Model file for the job. Use its own axes, mm. A direction names the side the tool comes from. Coordinates: 2 decimals unless noted, no trailing zeros. Write each loop counter-clockwise with the first axis right and the second up, starting at its lowest first coordinate (ties: lowest second). Pieces come first, ordered by that corner, then holes. Notation, with made-up numbers: M 27,-25.75 L 39,-25.75 A10 ccw 39,-9.75 Z; hole C 41.5,11 d7. An arc over 180 degrees is marked long. One line per question, with ' | ' between items. Start each with the question number.
(1) Two-plate mould, pull along Z, no slides. Class faces 1 (the face through (-0.423, 2.134, 6.778)), 2 (the face through (39, 19.05, 12)): +Z half, -Z half, draft (parallel to the pull), parting line (faces both ways), or undercut.
(2) Tool access for faces 3 (the face through (39, -19.05, 12)), 4 (the face through (17, -3.81, 1)), 5 (the face through (-13.247, 2.134, -0.143)): list every direction of +Z, -Z, +X, -X, +Y, -Y with a clear straight run to the whole face (end or side of a thin tool).
(3) Wall check: probe 1 along Z at (x, y) = (0, 0); probe 2 along Z at (x, y) = (0, 2). Give the ranges that are in metal, low to high.
(4) Flat gauge pins, fed straight in: pin 1 Ø4 at (x, z) = (0, -10) entering from -Y; pin 2 Ø3 at (x, y) = (41, 1) entering from -Z; pin 3 Ø6 at (x, z) = (0, 10) entering from +Y; pin 4 Ø2.5 at (x, z) = (10, 0) entering from +Y. Where does each tip first touch, or does it go through?
(5) Cut at D-D (x = -35.5). Write the cut outline in (y, z).
(6) Cut at A-A (z = 0). Count the separate pieces of the cut face and the enclosed holes in it, plus the area to 3 significant figures.
(7) Cut at C-C (y = 15.5). Write the cut outline in (x, z), plus the area to 3 significant figures.
(8) Cut at B-B (x = 10). Write the cut outline in (y, z), plus the area to 3 significant figures.
from build123d import *

# Parameters (mm, degrees)
SKETCH1_R                                           = 59.69
BOSS_EXTRUDE1_DEPTH                                 = 19.05
BOSS_EXTRUDE1_DEPTH_BACK                            = 19.05
SKETCH2_R                                           = 40.64
CUT_EXTRUDE2_DEPTH                                  = 15.24
SKETCH13_R                                          = 40.64
CUT_EXTRUDE7_DEPTH                                  = 15.24
SKETCH7_R                                           = 4
CUT_EXTRUDE6_DEPTH                                  = 25
SKETCH6_R                                           = 1.7
CUT_EXTRUDE5_DEPTH                                  = 10
CIRPATTERN2_COUNT                                   = 4
CBORE_FOR_M3_HEX_SOCKET_HEAD_CAP_SCREW1_D           = 3.4
CBORE_FOR_M3_HEX_SOCKET_HEAD_CAP_SCREW1_DEPTH       = 5
CBORE_FOR_M3_HEX_SOCKET_HEAD_CAP_SCREW1_CBORE_D     = 6.5
CBORE_FOR_M3_HEX_SOCKET_HEAD_CAP_SCREW1_CBORE_DEPTH = 3.4
CBORE_FOR_M3_HEX_SOCKET_HEAD_CAP_SCREW1_TIP         = 1.021463052
SKETCH14_R                                          = 15
CUT_EXTRUDE8_DEPTH                                  = 2


with BuildPart() as part:
    # Sketch1 → Boss-Extrude1 (new body, two sides)
    with BuildSketch(Plane(origin=(0, 0, 0), x_dir=(1, 0, 0), z_dir=(0, 1, 0))) as boss_extrude1_sk:
        Circle(SKETCH1_R)
    extrude(amount=BOSS_EXTRUDE1_DEPTH)
    extrude(boss_extrude1_sk.sketch, amount=-BOSS_EXTRUDE1_DEPTH_BACK)

    # Sketch2 → Cut-Extrude2 (cut)
    with BuildSketch(Plane.XZ.offset(19.05)):
        Circle(SKETCH2_R)
    extrude(amount=-CUT_EXTRUDE2_DEPTH, mode=Mode.SUBTRACT)

    # Sketch13 → Cut-Extrude7 (cut)
    with BuildSketch(Plane(origin=(0, 19.05, 0), x_dir=(1, 0, 0), z_dir=(0, 1, 0))):
        Circle(SKETCH13_R)
    extrude(amount=-CUT_EXTRUDE7_DEPTH, mode=Mode.SUBTRACT)

    # Sketch7 → Cut-Extrude6 (cut)
    with BuildSketch(Plane(origin=(0, 3.81, 0), x_dir=(1, 0, 0), z_dir=(0, 1, 0))):
        Circle(SKETCH7_R)
    cut_extrude6 = extrude(amount=-CUT_EXTRUDE6_DEPTH, mode=Mode.SUBTRACT)

    # Sketch6 → Cut-Extrude5 (cut)
    with BuildSketch(Plane(origin=(0, 3.81, 0), x_dir=(1, 0, 0), z_dir=(0, 1, 0))):
        with Locations((0, -10)):
            Circle(SKETCH6_R)
    cut_extrude5 = extrude(amount=-CUT_EXTRUDE5_DEPTH, mode=Mode.SUBTRACT)

    # CirPattern2: Cut-Extrude6, Cut-Extrude5 ×4 about axis
    cirpattern2_axis = Axis((0, 0, 0), (0, 1, 0))
    for i in range(1, CIRPATTERN2_COUNT):
        add(cut_extrude6.rotate(cirpattern2_axis, i * 360 / CIRPATTERN2_COUNT), mode=Mode.SUBTRACT)
        add(cut_extrude5.rotate(cirpattern2_axis, i * 360 / CIRPATTERN2_COUNT), mode=Mode.SUBTRACT)

    # CBORE for M3 Hex Socket Head Cap Screw1
    with Locations(Plane(origin=(0, 3.81, 0), x_dir=(1, 0, 0), z_dir=(0, 1, 0))):
        with Locations((0, -10), (10, 0), (0, 10), (-10, 0)):
            CounterBoreHole(CBORE_FOR_M3_HEX_SOCKET_HEAD_CAP_SCREW1_D / 2, CBORE_FOR_M3_HEX_SOCKET_HEAD_CAP_SCREW1_CBORE_D / 2, CBORE_FOR_M3_HEX_SOCKET_HEAD_CAP_SCREW1_CBORE_DEPTH, depth=CBORE_FOR_M3_HEX_SOCKET_HEAD_CAP_SCREW1_DEPTH)
            with Locations((0, 0, -(CBORE_FOR_M3_HEX_SOCKET_HEAD_CAP_SCREW1_DEPTH + CBORE_FOR_M3_HEX_SOCKET_HEAD_CAP_SCREW1_TIP / 2))):  # 118° drill point
                Cone(0, CBORE_FOR_M3_HEX_SOCKET_HEAD_CAP_SCREW1_D / 2, CBORE_FOR_M3_HEX_SOCKET_HEAD_CAP_SCREW1_TIP, mode=Mode.SUBTRACT)

    # Sketch14 → Cut-Extrude8 (cut)
    with BuildSketch(Plane.XZ.offset(3.81)):
        Circle(SKETCH14_R)
    extrude(amount=-CUT_EXTRUDE8_DEPTH, mode=Mode.SUBTRACT)


solid = part.part
Filled in:
1) face 1: undercut | face 2: draft
2) face 3: +Z, -Z, +X, -X, -Y | face 4: -Y | face 5: +Y
3) probe 1: -59.69 to -11.7, -8.3 to -4, 4 to 8.3, 11.7 to 59.69 | probe 2: -59.69 to -13.25, -6.75 to -4, 4 to 6.75, 13.25 to 59.69
4) pin 1: y = -1.81 | pin 2: z = -44.75 | pin 3: y = 0.41 | pin 4: through
5) outline: M -19.05,-47.99 L 19.05,-47.99 L 19.05,-19.78 L 3.81,-19.78 L 3.81,19.78 L 19.05,19.78 L 19.05,47.99 L -19.05,47.99 L -19.05,19.78 L -3.81,19.78 L -3.81,-19.78 L -19.05,-19.78 Z
6) separate pieces: 4 | enclosed holes: 0 | area: 1,910 mm²
7) outline: C 0,0 d119.38; hole C 0,0 d81.28 | area: 6,000 mm²
8) outline: M -19.05,-58.85 L 19.05,-58.85 L 19.05,-39.39 L 3.81,-39.39 L 3.81,-3.25 L 0.41,-3.25 L 0.41,-1.7 L -1.81,-1.7 L -1.81,-11.18 L -3.81,-11.18 L -3.81,-39.39 L -19.05,-39.39 Z; M -19.05,39.39 L -3.81,39.39 L -3.81,11.18 L -1.81,11.18 L -1.81,1.7 L 0.41,1.7 L 0.41,3.25 L 3.81,3.25 L 3.81,39.39 L 19.05,39.39 L 19.05,58.85 L -19.05,58.85 Z | area: 2,010 mm²
